```python
from build123d import *

# Parameters (mm, degrees)
AUFSATZ_LINEAR_AUSTRAGEN1_DEPTH = 10
SKIZZE2_R                       = 1.75
SCHNITT_LINEAR_AUSTRAGEN1_DEPTH = 38
SKIZZE4_R                       = 2.2
SCHNITT_LINEAR_AUSTRAGEN3_DEPTH = 52.2
VERRUNDUNG1_R                   = 10
SKIZZE5_W                       = 5.5
SKIZZE5_H                       = 5.5
SCHNITT_LINEAR_AUSTRAGEN4_DEPTH = 2
FASE1_SIZE                      = 1.5
SCHNITT_LINEAR_AUSTRAGEN5_DEPTH = 11


with BuildPart() as part:
    # Skizze1 → Aufsatz-Linear austragen1 (new body)
    with BuildSketch(Plane.XY):
        with BuildLine():
            Line((0.5, -28.495613698), (0.5, -32.496153619))
            Line((0.5, -32.496153619), (0.5, -39.496153619))
            Line((0.5, -39.496153619), (4.5, -39.496153619))
            Line((4.5, -39.496153619), (4.5, -32.186953879))
            ThreePointArc((4.5, -32.186953879), (31.590882714, -7.633225356), (18.7, 26.581196361))
            Line((18.7, 26.581196361), (18.7, 51.5))
            Line((18.7, 51.5), (10.2, 51.5))
            Line((10.2, 51.5), (10.2, 31.5))
            Line((10.2, 31.5), (-10.2, 31.5))
            Line((-10.2, 31.5), (-10.2, 51.5))
            Line((-10.2, 51.5), (-18.7, 51.5))
            Line((-18.7, 51.5), (-18.7, 26.581196361))
            ThreePointArc((-18.7, 26.581196361), (-31.590882714, -7.633225356), (-4.5, -32.186953879))
            Line((-4.5, -32.186953879), (-4.5, -39.496153619))
            Line((-4.5, -39.496153619), (-0.5, -39.496153619))
            Line((-0.5, -39.496153619), (-0.5, -32.496153619))
            Line((-0.5, -32.496153619), (-0.5, -28.495613698))
            ThreePointArc((-0.5, -28.495613698), (0, 28.5), (0.5, -28.495613698))
        make_face()
    extrude(amount=AUFSATZ_LINEAR_AUSTRAGEN1_DEPTH)

    # Skizze2 → Schnitt-Linear austragen1 (cut, through all)
    with BuildSketch(Plane.ZY.offset(4.5)):
        with Locations((5, -35.841553749)):
            Circle(SKIZZE2_R)
    extrude(amount=-SCHNITT_LINEAR_AUSTRAGEN1_DEPTH, mode=Mode.SUBTRACT)

    # Skizze4 → Schnitt-Linear austragen3 (cut, through all)
    with BuildSketch(Plane.ZY.offset(18.7)):
        with Locations((5, 41.5)):
            Circle(SKIZZE4_R)
    extrude(amount=-SCHNITT_LINEAR_AUSTRAGEN3_DEPTH, mode=Mode.SUBTRACT)

    # Verrundung1
    verrundung1_edges = [part.edges().sort_by_distance(p)[0] for p in [
        (-18.7, 26.581196361, 5),
        (18.7, 26.581196361, 5),
    ]]
    fillet(verrundung1_edges, radius=VERRUNDUNG1_R)

    # Skizze5 → Schnitt-Linear austragen4 (cut)
    with BuildSketch(Plane.ZY.offset(4.5)):
        with Locations((5, -35.841553749)):
            Rectangle(SKIZZE5_W, SKIZZE5_H)
    extrude(amount=-SCHNITT_LINEAR_AUSTRAGEN4_DEPTH, mode=Mode.SUBTRACT)

    # Fase1
    fase1_edges = [part.edges().sort_by_distance(p)[0] for p in [
        (-18.7, 41.422906559, 0),
        (31.036620275, -9.642520517, 0),
        (-18.7, 41.422906559, 10),
        (18.7, 41.422906559, 0),
        (18.7, 41.422906559, 10),
        (31.036620275, -9.642520517, 10),
        (-31.036620275, -9.642520517, 0),
        (-31.036620275, -9.642520517, 10),
        (19.547693958, 27.316508696, 0),
        (19.547693958, 27.316508696, 10),
        (-19.547693958, 27.316508696, 0),
        (-19.547693958, 27.316508696, 10),
    ]]
    chamfer(fase1_edges, length=FASE1_SIZE)

    # Skizze6 → Schnitt-Linear austragen5 (cut, through all)
    with BuildSketch(Plane.XY):
        Polygon((0, -82.914559746), (0, 27.830541285), (0.15, 27.830541285), (0.15, 32.208374164), (0, 32.208374164), (0, 82.914559746), (-62.169798489, 71.020337849), (-62.169798489, -54.918482242), align=None)
    extrude(amount=SCHNITT_LINEAR_AUSTRAGEN5_DEPTH, mode=Mode.SUBTRACT)


solid = part.part
```
Can you work these out from the model? Positions are in its coordinate system, mm. A direction names the side the tool comes from. Coordinates: 2 decimals unless noted, no trailing zeros. Order: outer loops, then holes, each group sorted by start corner. A loop starts at its lowest first (then second) coordinate and runs counter-clockwise, first axis right, second up. Notation, with made-up numbers: (-3.5, 28.5) -> (35.5, 28.5) arc R29 ccw to (35.5, 60.5) -> close; hole circle Ø10 at (-28.75, 69). An arc over 180 degrees is marked (long way). Write each question's results on one line, items separated by ' | '.
Item 1: I'm going to push flat-ended pins straight in: pin 1 Ø2.5 at (y, z) = (41.5, 5) entering from -X; pin 2 Ø2 at (x, y) = (19.5, 26.5) entering from -Z; pin 3 Ø5 at (y, z) = (-34, 4) entering from -X; pin 4 Ø5 at (y, z) = (43, 6) entering from -X. Where does each tip first touch, or does it pass through?
Results are:
pin 1: through | pin 2: z = 0.1 | pin 3: x = 0.5 | pin 4: x = 10.2
Item 2: I want a section at A-A, the plane y = 41.5. Write out the boundary of the cut face in (x, z), then the cut area to 4 significant figures.
Results are:
outline: (10.2, 0) -> (17.2, 0) -> (18.7, 1.5) -> (18.7, 2.8) -> (10.2, 2.8) -> close; (10.2, 7.2) -> (18.7, 7.2) -> (18.7, 8.5) -> (17.2, 10) -> (10.2, 10) -> close | area: 45.35 mm²
Item 3: I want a section at C-C, the plane y = 0. Write out the boundary of the cut face in (x, z).
Results are:
outline: (28.5, 0) -> (31, 0) -> (32.5, 1.5) -> (32.5, 8.5) -> (31, 10) -> (28.5, 10) -> close
Item 4: Which directions (+Z, -Z, +X, -X, +Y, -Y) give clear straight access to the entire face, cutting with the end or side of a thin tool? Please do faces 1 (the face through (18, 41.3, 0.8)), 2 (the face through (17.9, 41.3, 9.3)), 3 (the face through (10.2, 44, 5)).
Results are:
face 1: -Z, +X, +Y | face 2: +Z, +X, +Y | face 3: +Z, -Z, -X, +Y
Item 5: If I drill on line 1 along Y through (x, z) = (3.6, 5); line 2 along Y through (x, z) = (1.8, 5); line 3 along X through (y, z) = (46, 8.5), over which ranges is the centre line in solid material (lowest first)?
Results are:
line 1: -39.5 to -37.59, -34.09 to -28.27, 28.27 to 31.5 | line 2: -39.5 to -37.59, -34.09 to -28.44, 28.44 to 31.5 | line 3: 10.2 to 18.7
Item 6: If we mould it in two halves opening along Z, with no side actions, what happens to faces 4 (the face through (24, 16, 0)), 5 (the face through (30.88, -10.13, 4.95)), 6 (the face through (14.39, 39.352, 4.523)), 7 (the face through (2.47, -34.66, 3.71))? For each: +Z half, -Z half, draft (parallel to the pull), parting line (faces both ways), or undercut.
Results are:
face 4: -Z half | face 5: draft | face 6: undercut | face 7: undercut
Item 7: I want a section at D-D, the plane x = 11. Count the separate pieces of the cut face and the enclosed holes in it, then the cut area to 3 significant figures.
Results are:
separate pieces: 2 | enclosed holes: 1 | area: 277 mm²
